Model file for the job. Use its own axes, mm. Give positions to 0.01 mm unless a question says otherwise; leave off trailing zeros. Loops run counter-clockwise (first coordinate to the right, second up) from the corner with the lowest first, then second, coordinate; pieces in that order, holes last. Notation, with made-up numbers: M -19.75,26 L -12.75,26 A27 ccw -12.75,56 Z; hole C -14,-17 d6. An arc over 180 degrees is marked long. Answer in a Markdown table with one row per item.
```python
from build123d import *

# Parameters (mm, degrees)
SKETCH_1_W          = 74
SKETCH_1_H          = 35
EXTRUDE_1_DEPTH     = 3
SKETCH_3_R          = 1.55
CUT_EXTRUDE_1_DEPTH = 10
SKETCH_4_R          = 3.05
CUT_EXTRUDE_2_DEPTH = 10
SKETCH_5_R          = 11.5
CUT_EXTRUDE_3_DEPTH = 10


with BuildPart() as part:
    # 草图1 → 凸台-拉伸1 (new body)
    with BuildSketch(Plane(origin=(0, 0, 0), x_dir=(1, 0, 0), z_dir=(0, 1, 0))):
        Rectangle(SKETCH_1_W, SKETCH_1_H)
    extrude(amount=EXTRUDE_1_DEPTH)

    # 草图3 → 切除-拉伸1 (cut)
    with BuildSketch(Plane(origin=(0, 0, 0), x_dir=(-1, 0, 0), z_dir=(0, -1, 0))):
        with Locations(Location((13, -13, 0), (0, 0, 90))):
            Circle(SKETCH_3_R)
        with Locations(Location((-13, -13, 0), (0, 0, 90))):
            Circle(SKETCH_3_R)
        with Locations(Location((-13, 13, 0), (0, 0, 90))):
            Circle(SKETCH_3_R)
        with Locations(Location((13, 13, 0), (0, 0, 90))):
            Circle(SKETCH_3_R)
    extrude(amount=-CUT_EXTRUDE_1_DEPTH, mode=Mode.SUBTRACT)

    # 草图4 → 切除-拉伸2 (cut)
    with BuildSketch(Plane(origin=(0, 3, 0), x_dir=(1, 0, 0), z_dir=(0, 1, 0))):
        with Locations(Location((-27, 4, 0), (0, 0, 270))):
            Circle(SKETCH_4_R)
        with Locations(Location((27, 4, 0), (0, 0, 270))):
            Circle(SKETCH_4_R)
    extrude(amount=-CUT_EXTRUDE_2_DEPTH, mode=Mode.SUBTRACT)

    # 草图5 → 切除-拉伸3 (cut)
    with BuildSketch(Plane(origin=(0, 0, 0), x_dir=(-1, 0, 0), z_dir=(0, -1, 0))):
        with Locations(Location((0, 0, 0), (0, 0, 90))):
            Circle(SKETCH_5_R)
    extrude(amount=-CUT_EXTRUDE_3_DEPTH, mode=Mode.SUBTRACT)


solid = part.part
```
(1) Mould opens along Z. For faces 1 (the flat face through (-9, 3, -8)), 2 (the flat face through (-1, 1, 17.5)), 3 (the cylindrical face through (-12.93, 1.48, -11.45)) say: pulls with the +Z half, pulls with the -Z half, needs draft (parallel to the pull), parting line crosses it, or undercut.
Established:
| item | result |
|---|---|
| face 1 | needs draft |
| face 2 | pulls with the +Z half |
| face 3 | undercut |
(2) Saw through at C-C, the plane y = 2.25. Give the cut face in (x, z).
Established:
| item | result |
|---|---|
| outline | M -37,-17.5 L 37,-17.5 L 37,17.5 L -37,17.5 Z; hole C -27,-4 d6.1; hole C -13,-13 d3.1; hole C -13,13 d3.1; hole C 0,0 d23; hole C 13,-13 d3.1; hole C 13,13 d3.1; hole C 27,-4 d6.1 |
(3) Saw through at A-A, the plane x = 27. Give the cut face in (y, z).
Established:
| item | result |
|---|---|
| outline | M 0,-17.5 L 3,-17.5 L 3,-7.05 L 0,-7.05 Z; M 0,-0.95 L 3,-0.95 L 3,17.5 L 0,17.5 Z |
(4) Saw through at D-D, the plane z = -4. Give the cut face in (x, y).
Established:
| item | result |
|---|---|
| outline | M -37,0 L -30.05,0 L -30.05,3 L -37,3 Z; M -23.95,0 L -10.78,0 L -10.78,3 L -23.95,3 Z; M 10.78,0 L 23.95,0 L 23.95,3 L 10.78,3 Z; M 30.05,0 L 37,0 L 37,3 L 30.05,3 Z |
(5) Wall check: L1, parallel to X at y = 1.9, z = -13; L2, parallel to X at y = 1.35, z = 14; L3, parallel to X at y = 2.4, z = 0. Give the ranges that are in metal, low to high.
Established:
| item | result |
|---|---|
| L1 | x = -37 to -14.55, -11.45 to 11.45, 14.55 to 37 |
| L2 | x = -37 to -14.18, -11.82 to 11.82, 14.18 to 37 |
| L3 | x = -37 to -11.5, 11.5 to 37 |
(6) Saw through at B-B, the plane z = 13. Give the cut face in (x, y).
Established:
| item | result |
|---|---|
| outline | M -37,0 L -14.55,0 L -14.55,3 L -37,3 Z; M -11.45,0 L 11.45,0 L 11.45,3 L -11.45,3 Z; M 14.55,0 L 37,0 L 37,3 L 14.55,3 Z |
